Geometry check sheet. Reference: the model listing, model coordinates, mm. Coordinates: 2 decimals unless noted, no trailing zeros. Write each loop counter-clockwise with the first axis right and the second up, starting at its lowest first coordinate (ties: lowest second). Pieces come first, ordered by that corner, then holes. Notation, with made-up numbers: (-13.75, -2) -> (-5.75, -2) arc R26 cw to (-5.75, 37) -> close; hole circle Ø4 at (18, 20.25). An arc over 180 degrees is marked (long way). Put each result on its own line as item: value. Start each with the question number.
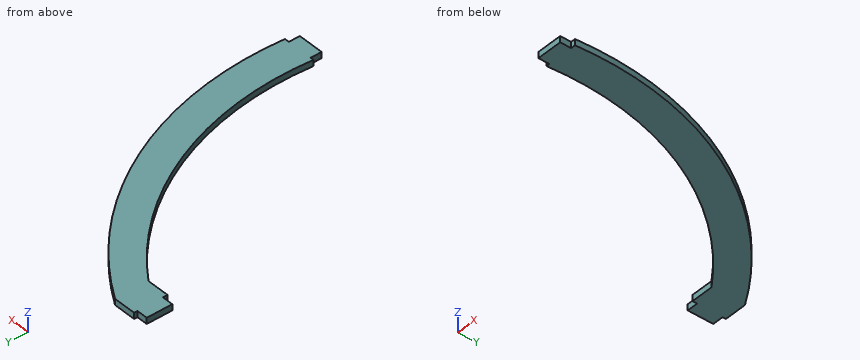
Autodesk Inventor part; units mm, degrees
ref_plane "YZ Plane" through (0, 0, 0) normal (1, 0, 0) x (0, 1, 0)
ref_plane "XZ Plane" through (0, 0, 0) normal (0, 1, 0) x (-1, 0, 0)
ref_plane "XY Plane" through (0, 0, 0) normal (0, 0, 1) x (1, 0, 0)
sketch "Sketch1" plane through (0, 0, 0) normal (0, 0, 1) x (1, 0, 0)
  line L0 (-6.985, -10.16) -> (6.985, -10.16)
  line L1 (5.08, -10.16) -> (5.08, -14.732)
  line L2 (5.08, -14.732) -> (-5.588, -14.732)
  line L3 (-5.588, -14.732) -> (-5.588, -10.16)
  line L4 (-68.0064, 116.8309) -> (-68.0064, 102.8609)
  line L5 (-68.0064, 104.7659) -> (-72.5784, 104.7659)
  line L6 (-72.5784, 104.7659) -> (-72.5784, 115.4339)
  line L7 (-72.5784, 115.4339) -> (-68.0064, 115.4339)
  line L8 (-68.0064, 116.8309) -> (-58.7093, 116.8309)
  arc A0 (6.985, -10.16) -> (-58.7093, 116.8309) centre (-125.8236, 1.6238) ccw
  line L9 (-68.0064, 102.8609) -> (-58.7093, 102.8609)
  arc A1 (-6.985, -10.16) -> (-58.7093, 102.8609) centre (-129.2297, 2.2407) ccw
  point P0 (0, 0)
  point P1 (0, -10.16)
  point P2 (-68.0064, 109.8459)
  dimension "d0" = 13.97
  dimension "d2" = 10.668
  dimension "d4" = 4.572
  dimension "d5" = 13.97
  dimension "d7" = 10.668
  dimension "d8" = 4.572
extrude "Extrusion1" add sketch "Sketch1" along normal blind 2.54
properties part number "RTS gift arm"
Item 1: Section check B-B, the plane x = -61. Enter the section's corners in (y, z).
Item 2: Scan lines: line 1 along Y through (x, z) = (-65.5, 1.9); line 2 along Y through (x, z) = (-68.5, 1.35); line 3 along X through (y, z) = (62, 0.7). Record each from-to range of solid material in increasing order. Write a range as [from, to].
Item 3: Section check C-C, the plane y = 60.5. Enter the section's corners in (x, z).
Item 4: Go/stop test with flat-tipped pins: P1, Ø0.8, axis at x = -71, z = 1.5, coming from the +Y side; P2, Ø0.6, axis at y = 104, z = 1, coming from the -X side; P3, Ø1.5, axis at x = -6.5, z = 1.5, coming from the -Y side; P4, Ø3, axis at x = -18, y = 83.5, coming from the +Z side. Record where each tip stops, or that it passes through.
Item 5: Section check A-A, the plane z = 0.9. Enter the section's corners in (x, y) (3 decimals), and give its area (3 significant figures).
From the geometry:
1. outline: (102.86, 0) -> (116.83, 0) -> (116.83, 2.54) -> (102.86, 2.54) -> close
2. line 1: [102.86, 116.83]
2. line 2: [104.77, 115.43]
2. line 3: [-21.87, -6.95]
3. outline: (-21.05, 0) -> (-6.2, 0) -> (-6.2, 2.54) -> (-21.05, 2.54) -> close
4. P1: y = 115.43
4. P2: x = -68.01
4. P3: y = -10.16
4. P4: through
5. outline: (-72.578, 104.766) -> (-68.006, 104.766) -> (-68.006, 102.861) -> (-58.709, 102.861) arc R122.872 cw to (-6.985, -10.16) -> (-5.588, -10.16) -> (-5.588, -14.732) -> (5.08, -14.732) -> (5.08, -10.16) -> (6.985, -10.16) arc R133.331 ccw to (-58.709, 116.831) -> (-68.006, 116.831) -> (-68.006, 115.434) -> (-72.578, 115.434) -> close
5. area: 2,070 mm²
